from build123d import *

# Parameters (mm, degrees)
SKETCH_1_W          = 112
SKETCH_1_H          = 117
EXTRUDE_1_DEPTH     = 30
FILLET_1_R          = 10
SKETCH_2_R          = 5
EXTRUDE_2_DEPTH     = 3
SKETCH_3_R          = 1.5
CUT_EXTRUDE_1_DEPTH = 5


with BuildPart() as part:
    # 草图1 → 凸台-拉伸1 (new body)
    with BuildSketch(Plane(origin=(0, 0, 0), x_dir=(1, 0, 0), z_dir=(0, 1, 0))):
        Rectangle(SKETCH_1_W, SKETCH_1_H)
    extrude(amount=EXTRUDE_1_DEPTH)

    # 圆角1
    fillet_1_edges = [part.edges().sort_by_distance(p)[0] for p in [
        (56, 15, 58.5),
        (-56, 15, 58.5),
        (-56, 15, -58.5),
        (56, 15, -58.5),
    ]]
    fillet(fillet_1_edges, radius=FILLET_1_R)

    # 草图2 → 凸台-拉伸2 (add)
    with BuildSketch(Plane(origin=(0, 30, 0), x_dir=(1, 0, 0), z_dir=(0, 1, 0))):
        with Locations(Location((-45.5, 47.5, 0), (0, 0, 90))):
            Circle(SKETCH_2_R)
        with Locations(Location((45.5, 47.5, 0), (0, 0, 90))):
            Circle(SKETCH_2_R)
        with Locations(Location((-45.5, -47.5, 0), (0, 0, 90))):
            Circle(SKETCH_2_R)
        with Locations(Location((45.5, -47.5, 0), (0, 0, 90))):
            Circle(SKETCH_2_R)
    extrude(amount=EXTRUDE_2_DEPTH)

    # 草图3 → 切除-拉伸1 (cut)
    with BuildSketch(Plane(origin=(0, 30, 0), x_dir=(1, 0, 0), z_dir=(0, 1, 0))):
        with Locations(Location((-42.5, 0, 0), (0, 0, 270))):
            Circle(SKETCH_3_R)
        with Locations(Location((42.5, 0, 0), (0, 0, 270))):
            Circle(SKETCH_3_R)
    extrude(amount=-CUT_EXTRUDE_1_DEPTH, mode=Mode.SUBTRACT)


solid = part.part
Check sheet for the modelled part. Datum: model origin and axes. Units: mm. A direction names the side the tool comes from. Give positions to 0.01 mm unless a question says otherwise; leave off trailing zeros. Order: outer loops, then holes, each group sorted by start corner. A loop starts at its lowest first (then second) coordinate and runs counter-clockwise, first axis right, second up. Notation, with made-up numbers: M 44,40 L 95,40 A20 ccw 95,48 Z; hole C 52,60 d11. An arc over 180 degrees is marked long. Answer as CSV lines item,"result". Start each with the question number.
Item 1: Cross-section at A-A on z = 0. Enter the section's corners in (x, y).
Item 2: Thickness scan on line 1 (X direction, y = 26, z = 0); line 2 (Y direction, x = -40, z = -36); line 3 (Z direction, x = -42, y = 27). Record the ranges inside material, lowest first. Write a range as [from, to].
Item 3: Tool access check on faces 1 (the face through (41, 28, 0)), 2 (the face through (-1, 0, -1)). Record the directions out of +Z, -Z, +X, -X, +Y, -Y that give a thin tool (end or side, any length) a straight path to the whole face; none if there is none.
Item 4: Cross-section at B-B on x = -42.5. Enter the section's corners in (y, z).
Item 5: Cross-section at C-C on x = 48.5. Enter the section's corners in (y, z).
Item 6: Gauge pin test, flat end, axial feed: P1, Ø2.5, axis at x = -42, z = 0, coming from the +Y side. Record the tip position at first contact, or that the pin passes through.
Item 7: Cross-section at D-D on z = 23. Enter the section's corners in (x, y), plus the area to 3 significant figures.
Item 8: Mould release check, pull along X, two halves, no side actions. Record for faces 3 (the face through (43, 25, 0)), 4 (the face through (-48.879, 31.479, -43.815)), 5 (the face through (-46, 33, 48)), 6 (the face through (52.99, 15.21, 55.65)): +X half, -X half, draft (parallel to the pull), parting line (faces both ways), or undercut.
Established:
1,outline,"M -56,0 L 56,0 L 56,30 L 44,30 L 44,25 L 41,25 L 41,30 L -41,30 L -41,25 L -44,25 L -44,30 L -56,30 Z"
2,line 1,"x = [-56, -44], [-41, 41], [44, 56]"
2,line 2,"y = [0, 30]"
2,line 3,"z = [-58.5, -1.41], [1.41, 58.5]"
3,face 1,"+Y"
3,face 2,"+Z, -Z, +X, -X, -Y"
4,outline,"M 0,-58.5 L 30,-58.5 L 30,-51.5 L 33,-51.5 L 33,-43.5 L 30,-43.5 L 30,-1.5 L 25,-1.5 L 25,1.5 L 30,1.5 L 30,43.5 L 33,43.5 L 33,51.5 L 30,51.5 L 30,58.5 L 0,58.5 Z"
5,outline,"M 0,-58.18 L 30,-58.18 L 30,-51.5 L 33,-51.5 L 33,-43.5 L 30,-43.5 L 30,43.5 L 33,43.5 L 33,51.5 L 30,51.5 L 30,58.18 L 0,58.18 Z"
6,P1,"stops at y = 30"
7,outline,"M -56,0 L 56,0 L 56,30 L -56,30 Z"
7,area,"3,360 mm^2"
8,face 3,"undercut"
8,face 4,"undercut"
8,face 5,"draft"
8,face 6,"+X half"
